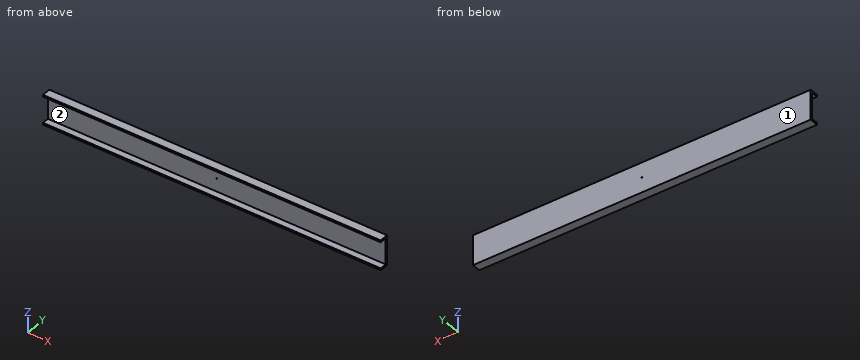
from build123d import *

# Parameters (mm, degrees)
F0_R     = 0.5
F1_DEPTH = 2
F2_W     = 350
F2_H     = 2
F3_DEPTH = 7
F6_DEPTH = 2


with BuildPart() as f1:
    # F0 (on Front) → F1 (new body)
    with BuildSketch(Plane.XZ):
        Polygon((175, 13.5), (-175, 13.5), (-175, 11.5), (-175, -15.5), (-175, -17.5), (175, -17.5), (175, -15.5), (175, 11.5), align=None)
        with Locations((0, -2)):
            Circle(F0_R, mode=Mode.SUBTRACT)
    extrude(amount=F1_DEPTH)

    # F2 (on face) → F3 (join)
    with BuildSketch(Plane.XZ.offset(2)):
        with Locations((0, 12.5)):
            Rectangle(F2_W, F2_H)
        with Locations((0, -16.5)):
            Rectangle(F2_W, F2_H)
    extrude(amount=F3_DEPTH)

    # F0 (on Front) → F6 (cut)
    with BuildSketch(Plane.XZ):
        Polygon((175, 13.5), (-175, 13.5), (-175, 11.5), (-175, -15.5), (-175, -17.5), (175, -17.5), (175, -15.5), (175, 11.5), align=None)
        with Locations((0, -2)):
            Circle(F0_R, mode=Mode.SUBTRACT)
    extrude(amount=-F6_DEPTH, mode=Mode.SUBTRACT)


with BuildPart() as f4_1:
    # F4: copy of F1
    add(f1.part)


solid = f1.part
Model file for the job. Use its own axes, mm. Face numbers are marked on the shaded views. Give positions to 0.01 mm unless a question says otherwise; leave off trailing zeros. Order: outer loops, then holes, each group sorted by start corner. A loop starts at its lowest first (then second) coordinate and runs counter-clockwise, first axis right, second up. Notation, with made-up numbers: (27.25, -26.5) - (33.25, -26.5) arc R25 cw to (33.25, -11.5) - close; hole circle Ø7 at (-19, -5.75). An arc over 180 degrees is marked (long way). One line per item, written item: value.
Item 1: Slice it at A-A (y = -7.25). List the corners of the cut face in (x, z), then the cut area to 3 significant figures.
Response values:
outline: (-175, -17.5) - (175, -17.5) - (175, -15.5) - (-175, -15.5) - close; (-175, 11.5) - (175, 11.5) - (175, 13.5) - (-175, 13.5) - close
area: 1,400 mm2
Item 2: Two-plate mould, pull along Z, no slides. Class the marked faces 1 and 2: released by +Z, released by -Z, zero draft, split by the parting line, or undercut.
Response values:
face 1: zero draft
face 2: undercut
Item 3: Wall check: line 1 (Z direction, x = 35, y = -2.25); line 2 (Z direction, x = 0, y = -0.45); line 3 (Y direction, x = -34, z = -4). Give the ranges that are in metal, low to high.
Response values:
line 1: -17.5 to -15.5, 11.5 to 13.5
line 2: -17.5 to -2.5, -1.5 to 13.5
line 3: -2 to 0
Item 4: Slice it at B-B (x = -104). List the corners of the cut face in (y, z).
Response values:
outline: (-9, -17.5) - (0, -17.5) - (0, 13.5) - (-9, 13.5) - (-9, 11.5) - (-2, 11.5) - (-2, -15.5) - (-9, -15.5) - close
Item 5: Pin check, flat tip, straight feed: pin 1 Ø2 at (x, z) = (96, 8) entering from -Y. Stop position of the tip, or through.
Response values:
pin 1: y = -2
